Design review of the part built by this model. Coordinates are the model's own, in mm. Face numbers are marked on the shaded views. A direction names the side the tool comes from. Round coordinates to 2 decimals unless told otherwise and drop trailing zeros. Order: outer loops, then holes, each group sorted by start corner. A loop starts at its lowest first (then second) coordinate and runs counter-clockwise, first axis right, second up. Notation, with made-up numbers: (-8, -7) - (36, -7) arc R14 ccw to (36, 20) - close; hole circle Ø10 at (45.25, 1). An arc over 180 degrees is marked (long way). Answer as a JSON object with one key per item and string values. Group by question number.
from build123d import *

# Parameters (mm, degrees)
BOSS_EXTRUDE1_DEPTH = 2
BOSS_EXTRUDE2_DEPTH = 14
SKETCH3_R           = 0.8
CUT_EXTRUDE1_DEPTH  = 17.763054614
SKETCH4_R           = 6
BOSS_EXTRUDE3_DEPTH = 12


with BuildPart() as part:
    # Sketch1 → Boss-Extrude1 (new body)
    with BuildSketch(Plane(origin=(0, 0, 0), x_dir=(1, 0, 0), z_dir=(0, 1, 0))):
        with BuildLine():
            Line((-6.5, 7), (6.5, 7))
            ThreePointArc((6.5, 7), (6.853553391, 6.853553391), (7, 6.5))
            Line((7, 6.5), (7, -6.5))
            ThreePointArc((7, -6.5), (6.853553391, -6.853553391), (6.5, -7))
            Line((6.5, -7), (-6.5, -7))
            ThreePointArc((-6.5, -7), (-6.853553391, -6.853553391), (-7, -6.5))
            Line((-7, -6.5), (-7, 6.5))
            ThreePointArc((-7, 6.5), (-6.853553391, 6.853553391), (-6.5, 7))
        make_face()
    extrude(amount=BOSS_EXTRUDE1_DEPTH)

    # Sketch2 → Boss-Extrude2 (add, through all)
    with BuildSketch(Plane.ZY.offset(7)):
        with BuildLine():
            Line((-1.5, 4.5), (-1.5, 2))
            Line((-1.5, 2), (1.5, 2))
            Line((1.5, 2), (1.5, 4.5))
            ThreePointArc((1.5, 4.5), (0, 6), (-1.5, 4.5))
        make_face()
    extrude(amount=-BOSS_EXTRUDE2_DEPTH)

    # Sketch3 → Cut-Extrude1 (cut, through all)
    with BuildSketch(Plane.ZY.offset(7)):
        with Locations((0, 4.5)):
            Circle(SKETCH3_R)
    extrude(amount=-CUT_EXTRUDE1_DEPTH, mode=Mode.SUBTRACT)

    # Sketch4 → Boss-Extrude3 (add)
    with BuildSketch(Plane(origin=(0, 2, 0), x_dir=(1, 0, 0), z_dir=(0, 1, 0))):
        with Locations(Location((0, 0, 0), (0, 0, 165.522487814))):
            Circle(SKETCH4_R)
    extrude(amount=BOSS_EXTRUDE3_DEPTH)


solid = part.part
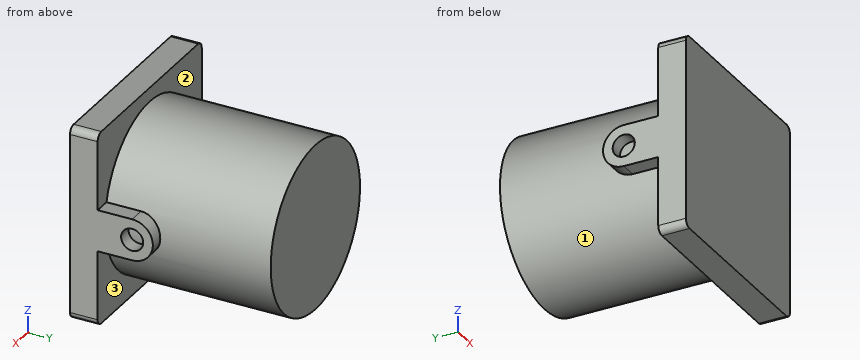
1. Clearance check with flat-ended pins moving along their axes: P1, Ø3, axis at y = 6.5, z = 4.5, coming from the +X side; P2, Ø0.6, axis at x = -6.5, y = 3, coming from the +Z side; P3, Ø2, axis at y = 4.5, z = 0, coming from the -X side; P4, Ø1.3, axis at y = 4.5, z = 0, coming from the -X side. State where each tip first meets the part, or that it passes through.
2. To check wall thickness, follow line 1 (Z direction, x = -6.6, y = 4.5); line 2 (Y direction, x = -6.4, z = 0); line 3 (X direction, y = 7.25, z = 0). State the ranges of each line that lie inside material, in increasing order. Write a range as from..to.
3. Take a section at B-B, the plane y = 2.75. Give the boundary of the cut face in (x, z).
4. Take a section at A-A, the plane z = 0. Give the boundary of the cut face in (x, y).
5. Tool access review of the marked faces 1, 2 and 3: name each direction out of +Z, -Z, +X, -X, +Y, -Y from which nothing blocks a thin tool from reaching the whole face with its end or side.
6. Take a section at C-C, the plane x = 0. Give the boundary of the cut face in (y, z), then the cut area to 3 significant figures.
Response values:
{
 "1": {"P1": "x = 5.2", "P2": "z = 1.5", "P3": "x = -7", "P4": "x = -6"},
 "2": {"line 1": "-1.5..-0.8, 0.8..1.5", "line 2": "0..3.7, 5.3..6", "line 3": "-6..6"},
 "3": {"outline": "(-7, -1.5) - (-5.81, -1.5) arc R6 ccw to (5.81, -1.5) - (7, -1.5) - (7, 1.5) - (5.81, 1.5) arc R6 ccw to (-5.81, 1.5) - (-7, 1.5) - close"},
 "4": {"outline": "(-7, 0) - (7, 0) - (7, 3.7) - (6, 3.7) - (6, 5.3) - (7, 5.3) - (7, 6) - (6, 6) - (6, 14) - (-6, 14) - (-6, 6) - (-7, 6) - (-7, 5.3) - (-6, 5.3) - (-6, 3.7) - (-7, 3.7) - close"},
 "5": {"face 1": "+Y", "face 2": "+Z, +Y", "face 3": "-Z, +Y"},
 "6": {"outline": "(0, -7) - (2, -7) - (2, -6) - (14, -6) - (14, 6) - (2, 6) - (2, 7) - (0, 7) - close", "area": "172 mm2"}
}
